Autodesk Inventor part; units mm, degrees
ref_plane "YZ Plane" through (0, 0, 0) normal (1, 0, 0) x (0, 1, 0)
ref_plane "XZ Plane" through (0, 0, 0) normal (0, 1, 0) x (-1, 0, 0)
ref_plane "XY Plane" through (0, 0, 0) normal (0, 0, 1) x (1, 0, 0)
sketch "Sketch1" plane through (0, 0, 0) normal (0, 1, 0) x (-1, 0, 0)
  circle A0 centre (0, 0) radius 2.8
  circle A1 centre (0, 0) radius 7.5
  dimension "d0" = 5.6
  dimension "d1" = 15
extrude "Extrusion1" add sketch "Sketch1" along normal blind 7.25
sketch "Sketch2" plane through (0, 7.25, 0) normal (0, 1, 0) x (1, 0, 0)
  circle A0 centre (0, 0) radius 4.5
  circle A1 centre (0, 0) radius 2.8
  dimension "d4" = 9
extrude "Extrusion2" add sketch "Sketch2" along normal blind 0.75
chamfer "Chamfer1" distance 1 angle 45 1 edges at (7.5, 7.25, 0)
properties part number "Y-Carraige_Spacer_LM3044" material "ABS Plastic"
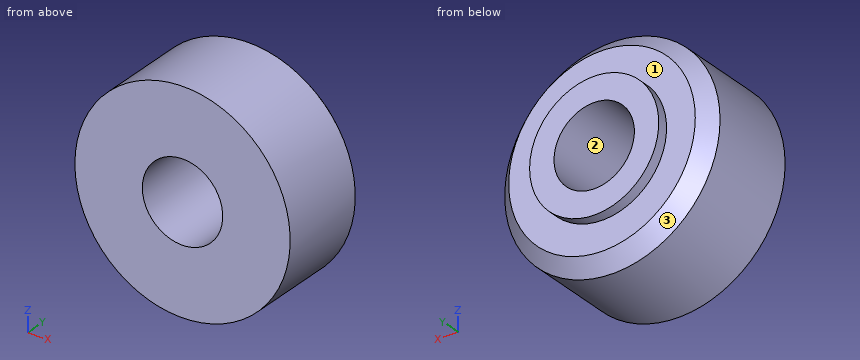
Geometry: final body of the model. Coordinates: model frame, mm. Face numbers are marked on the shaded views. Round coordinates to 2 decimals unless told otherwise and drop trailing zeros. Loops run counter-clockwise (first coordinate to the right, second up) from the corner with the lowest first, then second, coordinate; pieces in that order, holes last.
Item 1: Mould query, pull axis Z, two halves, no side actions, for the marked faces 1, 2 and 3. Classes: released by +Z, released by -Z, zero draft, split by the parting line, or undercut.
Checked values:
face 1: zero draft
face 2: undercut
face 3: split by the parting line
Item 2: Section B-B, the plane y = 1.5. Output: boundary loops of the cut face in (x, z), plus the area to 3 significant figures.
Checked values:
outline: circle Ø15 at (0, 0); hole circle Ø5.6 at (0, 0)
area: 152 mm2
Item 3: Line query: L1, parallel to Z at x = 0, y = 3.25; L2, parallel to Y at x = 0.75, z = -6; L3, parallel to Z at x = 0.75, y = 6.5. Output: solid intervals per line, ascending.
Checked values:
L1: z = -7.5 to -2.8, 2.8 to 7.5
L2: y = 0 to 7.25
L3: z = -7.21 to -2.7, 2.7 to 7.21
Item 4: Contact query for flat-ended pins moving along their axis: P1, Ø1.5, axis at x = 1.5, y = 5, coming from the -Z side; P2, Ø3, axis at x = 5.5, y = 2.5, coming from the -Z side. Output: stop coordinate, or through.
Checked values:
P1: stops at z = -7.46
P2: stops at z = -6.34
